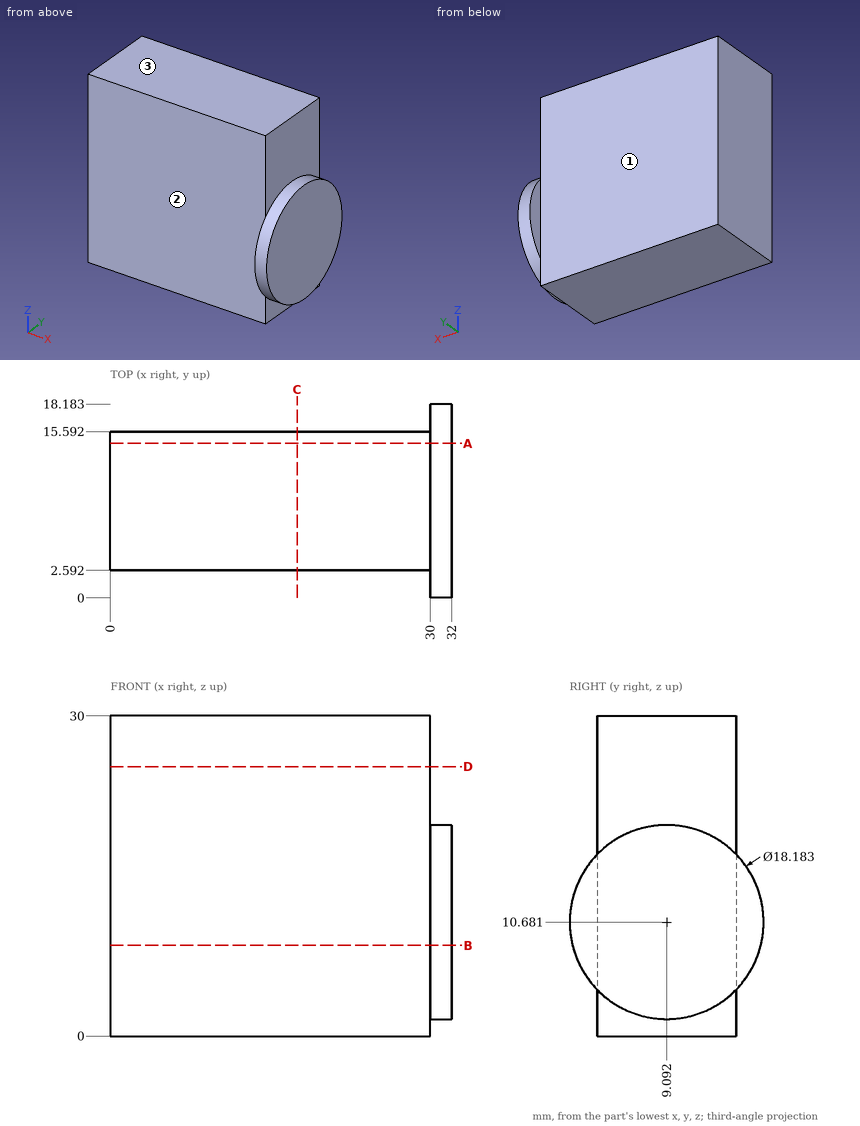
Geometry: see drawing. Coordinates: mm, zero at the bounding-box minimum. A direction names the side the tool comes from. Give positions to 0.01 mm unless a question says otherwise; leave off trailing zeros. Order: outer loops, then holes, each group sorted by start corner. A loop starts at its lowest first (then second) coordinate and runs counter-clockwise, first axis right, second up. Notation, with made-up numbers: (-15, -1.5) -> (-9, -1.5) arc R20 cw to (-9, 31.5) -> close; hole circle Ø3 at (85, -0.75). An arc over 180 degrees is marked (long way). Write each question's results on one line, items separated by ' | '. Start each with the question number.
1) Line query: line 1 (Y direction, x = 16, z = 14); line 2 (X direction, y = 12, z = 24); line 3 (X direction, y = 0.5, z = 9.5). Output: solid intervals per line, ascending. Write a range as from..to.
2) Set-up query: the marked faces 1, 2 and 3. Return all of +Z, -Z, +X, -X, +Y, -Y with unobstructed straight access to the full face (end or side cutting, diameter ignored); none if empty.
3) Section C-C (x = 17.5). Return loops of the section in (y, z), then the cut area to 3 significant figures.
4) Section B-B (z = 8.5). Return loops of the section in (x, y) (1 decimal), then the cut area to 3 significant figures.
5) First-contact query: pin 1 (4 mm diameter, centred on x = 26.5, z = 18.5, fed in from +Y); pin 2 (3 mm diameter, centred on x = 23, z = 6, fed in from -Y); pin 3 (0.8 mm diameter, centred on y = 17, z = 13.5, fed in from -X). Flat tips, straight axial feed; report the tip coordinate or a pass-through.
6) Section D-D (z = 25.25). Return loops of the section in (x, y), then the cut area to 3 significant figures.
7) Section A-A (y = 14.5). Return loops of the section in (x, z).
Calculated:
1) line 1: 2.59..15.59 | line 2: 0..30 | line 3: 30..32
2) face 1: +Z, -Z, -X, +Y | face 2: +Z, -Z, -X, -Y | face 3: +Z, +X, -X, +Y, -Y
3) outline: (2.59, 0) -> (15.59, 0) -> (15.59, 30) -> (2.59, 30) -> close | area: 390 mm2
4) outline: (0, 2.6) -> (30, 2.6) -> (30, 0.3) -> (32, 0.3) -> (32, 17.9) -> (30, 17.9) -> (30, 15.6) -> (0, 15.6) -> close | area: 425 mm2
5) pin 1: y = 15.59 | pin 2: y = 2.59 | pin 3: x = 30
6) outline: (0, 2.59) -> (30, 2.59) -> (30, 15.59) -> (0, 15.59) -> close | area: 390 mm2
7) outline: (0, 0) -> (30, 0) -> (30, 3.37) -> (32, 3.37) -> (32, 17.99) -> (30, 17.99) -> (30, 30) -> (0, 30) -> close
